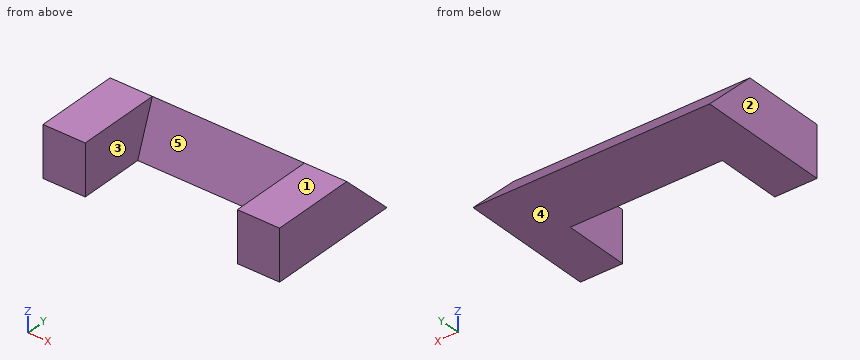
from build123d import *

# Parameters (mm, degrees)
SKETCH1_W             = 25
SKETCH1_H             = 30
BOSS_EXTRUDE1_DEPTH   = 50
BOSS_EXTRUDE1_2_DEPTH = 50
BOSS_EXTRUDE2_START   = -140
BOSS_EXTRUDE2_DEPTH   = 140
BOSS_EXTRUDE3_DEPTH   = 90


with BuildPart() as part:
    # Sketch1 → Boss-Extrude1 (new body)
    with BuildSketch(Plane(origin=(0, 0, 0), x_dir=(1, 0, 0), z_dir=(0, 1, 0))):
        with Locations((-31.032110092, 2.339449541)):
            Rectangle(SKETCH1_W, SKETCH1_H)
    extrude(amount=BOSS_EXTRUDE1_DEPTH)



with BuildPart() as body_2:
    # Sketch1 → Boss-Extrude1 2 (new body)
    with BuildSketch(Plane(origin=(0, 0, 0), x_dir=(1, 0, 0), z_dir=(0, 1, 0))):
        with Locations((83.967889908, 2.339449541)):
            Rectangle(SKETCH1_W, SKETCH1_H)
    extrude(amount=BOSS_EXTRUDE1_2_DEPTH)


with BuildPart() as part_1:
    add(part.part)

    add(body_2.part)  # Boss-Extrude2 merges body 2
    # Sketch2 → Boss-Extrude2 (add)
    with BuildSketch(Plane(origin=(96.467889908, 0, 0), x_dir=(0, 0, -1), z_dir=(1, 0, 0)).offset(BOSS_EXTRUDE2_START)):
        Polygon((-12.660550459, 50), (17.339449541, 50), (17.339449541, 80), align=None)
    extrude(amount=BOSS_EXTRUDE2_DEPTH)

    # Sketch3 → Boss-Extrude3 (add)
    with BuildSketch(Plane(origin=(-18.532110092, 0, 0), x_dir=(0, 0, -1), z_dir=(1, 0, 0))):
        Polygon((-12.660550459, 50), (17.339449541, 39.080892972), (17.339449541, 50), align=None)
    extrude(amount=BOSS_EXTRUDE3_DEPTH)


solid = part_1.part
Model file for the job. Use its own axes, mm. Face numbers are marked on the shaded views. A direction names the side the tool comes from. Give positions to 0.01 mm unless a question says otherwise; leave off trailing zeros. Write each loop counter-clockwise with the first axis right and the second up, starting at its lowest first coordinate (ties: lowest second). Pieces come first, ordered by that corner, then holes. Notation, with made-up numbers: M 24,88.25 L 47,88.25 A20 cw 47,93.25 Z; hole C 32.5,8.5 d3. An arc over 180 degrees is marked long. One line per item, written item: value. Start each with the question number.
Q1. Probe probe 1 along X at (y, z) = (39, 2); probe 2 along Y at (x, z) = (-16, -12); probe 3 along Z at (x, y) = (68, 63). List the from-to ranges inside material, lowest first. Write a range as [from, to].
Q2. Saw through at A-A, the plane y = 29.5. Write the cut outline in (x, z), plus the area to 3 significant figures.
Q3. Two-plate mould, pull along X, no slides. Class the marked faces 1, 2 and 3: +X half, -X half, draft (parallel to the pull), parting line (faces both ways), or undercut.
Q4. Saw through at D-D, the plane y = 72. Write the cut outline in (x, z).
Q5. Saw through at B-B, the plane z = -14. Write the cut outline in (x, y).
Q6. Drop flat-ended pins along their axis: pin 1 Ø12 at (y, z) = (69.5, 5.5) entering from -X; pin 2 Ø4 at (x, z) = (67.5, 9) entering from +Y; pin 3 Ø10 at (x, z) = (25, 7) entering from -Y. Give the stop position or say it passes through.
Q7. 3-axis set-ups, long thin cutter, end or side, ignore diameter. For the marked faces 4 and 5: which of +Z, -Z, +X, -X, +Y, -Y reach the whole face in a straight line?
Q8. Saw through at C-C, the plane x = -25. Write the cut outline in (y, z).
Output values:
1. probe 1: x = [-43.53, -18.53], [71.47, 96.47]
1. probe 2: y = [41.02, 74.66]
1. probe 3: z = [-17.34, -0.34]
2. outline: M -43.53,-17.34 L -18.53,-17.34 L -18.53,12.66 L -43.53,12.66 Z; M 71.47,-17.34 L 96.47,-17.34 L 96.47,12.66 L 71.47,12.66 Z
2. area: 1,500 mm²
3. face 1: draft
3. face 2: -X half
3. face 3: undercut
4. outline: M -43.53,-17.34 L 96.47,-17.34 L 96.47,-9.34 L -43.53,-9.34 Z
5. outline: M -43.53,0 L -18.53,0 L -18.53,40.3 L 71.47,40.3 L 71.47,0 L 96.47,0 L 96.47,76.66 L -43.53,76.66 Z
6. pin 1: passes through
6. pin 2: stops at y = 55.66
6. pin 3: stops at y = 46.12
7. face 4: -Z, +X, -X, +Y, -Y
7. face 5: +Z, -Y
8. outline: M 0,-17.34 L 80,-17.34 L 50,12.66 L 0,12.66 Z
